The model under review builds one solid part; all positions refer to its coordinate system, in mm. A direction names the side the tool comes from. Round coordinates to 2 decimals unless told otherwise and drop trailing zeros. Write each loop counter-clockwise with the first axis right and the second up, starting at its lowest first coordinate (ties: lowest second). Pieces come first, ordered by that corner, then holes. Notation, with made-up numbers: (-35.5, 85.5) - (18.5, 85.5) arc R26 ccw to (18.5, 115.5) - close; hole circle Ø5 at (-9, -22). An arc over 180 degrees is marked (long way). Use one line per item in the form item = value.
Autodesk Inventor part; units mm, degrees
ref_plane "YZ Plane" through (0, 0, 0) normal (1, 0, 0) x (0, 1, 0)
ref_plane "XZ Plane" through (0, 0, 0) normal (0, 1, 0) x (-1, 0, 0)
ref_plane "XY Plane" through (0, 0, 0) normal (0, 0, 1) x (1, 0, 0)
sketch "Sketch2" plane through (0, 0, 0) normal (1, 0, 0) x (0, 1, 0)
  arc A0 (12.5, 50.9902) -> (-12.5, 50.9902) centre (0, 0) ccw
  arc A1 (-19.5, 39.443) -> (-17.7114, 42.7254) centre (-20.9403, 42.3564) ccw
  line L0 (-17.7114, 42.7254) -> (-17.7881, 43.3968)
  arc A2 (-12.5, 50.9902) -> (-17.7881, 43.3968) centre (-10.8333, 44.1915) ccw
  line L1 (0, 0) -> (0, 52.5) construction
  arc A3 (17.7114, 42.7254) -> (19.5, 39.443) centre (20.9403, 42.3564) ccw
  line L2 (17.7114, 42.7254) -> (17.7881, 43.3968)
  arc A4 (17.7881, 43.3968) -> (12.5, 50.9902) centre (10.8333, 44.1915) ccw
  arc A5 (-44.6318, 27.645) -> (-52.3573, 3.8686) centre (0, 0) ccw
  arc A6 (-43.5384, -6.357) -> (-46.1074, -3.6416) centre (-46.7543, -6.8266) ccw
  line L3 (-46.1074, -3.6416) -> (-46.7696, -3.5071)
  arc A7 (-52.3573, 3.8686) -> (-46.7696, -3.5071) centre (-45.3763, 3.3528) ccw
  line L4 (0, 0) -> (-49.9305, 16.2234) construction
  arc A8 (-35.776, 30.3278) -> (-44.6318, 27.645) centre (-38.6809, 23.959) ccw
  line L5 (-35.1611, 30.0474) -> (-35.776, 30.3278)
  arc A9 (-35.1611, 30.0474) -> (-31.4867, 30.7342) centre (-33.8124, 33.0043) ccw
  arc A10 (-40.084, -33.9046) -> (-19.8586, -48.5993) centre (0, 0) ccw
  arc A11 (-7.4082, -43.3719) -> (-10.7846, -44.976) centre (-7.9554, -46.5755) ccw
  line L6 (-10.7846, -44.976) -> (-11.1171, -45.5643)
  arc A12 (-19.8586, -48.5993) -> (-11.1171, -45.5643) centre (-17.2108, -42.1194) ccw
  line L7 (0, 0) -> (-30.8587, -42.4734) construction
  arc A13 (-39.8989, -24.6532) -> (-40.084, -33.9046) centre (-34.7395, -29.384) ccw
  line L8 (-39.4421, -24.1551) -> (-39.8989, -24.6532)
  arc A14 (-39.4421, -24.1551) -> (-38.9598, -20.4482) centre (-41.8376, -21.9586) ccw
  arc A15 (19.8586, -48.5993) -> (40.084, -33.9046) centre (0, 0) ccw
  arc A16 (38.9598, -20.4482) -> (39.4421, -24.1551) centre (41.8376, -21.9586) ccw
  line L9 (39.4421, -24.1551) -> (39.8989, -24.6532)
  arc A17 (40.084, -33.9046) -> (39.8989, -24.6532) centre (34.7395, -29.384) ccw
  line L10 (0, 0) -> (30.8587, -42.4734) construction
  arc A18 (11.1171, -45.5643) -> (19.8586, -48.5993) centre (17.2108, -42.1194) ccw
  line L11 (10.7846, -44.976) -> (11.1171, -45.5643)
  arc A19 (10.7846, -44.976) -> (7.4082, -43.3719) centre (7.9554, -46.5755) ccw
  arc A20 (52.3573, 3.8686) -> (44.6318, 27.645) centre (0, 0) ccw
  arc A21 (31.4867, 30.7342) -> (35.1611, 30.0474) centre (33.8124, 33.0043) ccw
  line L12 (35.1611, 30.0474) -> (35.776, 30.3278)
  arc A22 (44.6318, 27.645) -> (35.776, 30.3278) centre (38.6809, 23.959) ccw
  line L13 (0, 0) -> (49.9305, 16.2234) construction
  arc A23 (46.7696, -3.5071) -> (52.3573, 3.8686) centre (45.3763, 3.3528) ccw
  line L14 (46.1074, -3.6416) -> (46.7696, -3.5071)
  arc A24 (46.1074, -3.6416) -> (43.5384, -6.357) centre (46.7543, -6.8266) ccw
  arc A25 (38.9598, -20.4482) -> (43.5384, -6.357) centre (0, 0) ccw
  arc A26 (-7.4082, -43.3719) -> (7.4082, -43.3719) centre (0, 0) ccw
  arc A27 (-43.5384, -6.357) -> (-38.9598, -20.4482) centre (0, 0) ccw
  arc A28 (31.4867, 30.7342) -> (19.5, 39.443) centre (0, 0) ccw
  arc A29 (-19.5, 39.443) -> (-31.4867, 30.7342) centre (0, 0) ccw
  dimension "d75" = 52.5
  dimension "d76" = 7
  dimension "d77" = 3.25
  dimension "d80" = 360
  dimension "d83" = 44
  dimension "d84" = 12.5
  dimension "d85" = 19.5
extrude "Extrusion1" add sketch "Sketch2" along normal blind 5
sketch "Sketch3" plane through (0, 0, 0) normal (-1, 0, 0) x (0, 0, 1)
  circle A0 centre (0, 0) radius 11.5
  circle A1 centre (0, 0) radius 9
  point P0 (0, 0)
  dimension "d55" = 23
  dimension "d56" = 18
extrude "Extrusion2" add sketch "Sketch3" along normal blind 27.81
fillet "Fillet1" radius 14 1 edges at (0, 0, -11.5)
sketch "Sketch4" plane through (5, 0, 0) normal (1, 0, 0) x (0, 0, -1)
  circle A0 centre (0, 0) radius 32.5
  point P0 (0, 0)
  dimension "d60" = 65
extrude "Extrusion3" add sketch "Sketch4" along normal blind 5
sketch "Sketch5" plane through (10, 0, 0) normal (1, 0, 0) x (0, 0, -1)
  circle A0 centre (0, 0) radius 13
  point P0 (0, 0)
  dimension "d63" = 26
extrude "Extrusion4" add sketch "Sketch5" along normal blind 3.108
sketch "Sketch6" plane through (13.108, 0, 0) normal (1, 0, 0) x (0, 0, -1)
  circle A0 centre (0, 0) radius 9
  point P0 (0, 0)
extrude "Extrusion5" cut sketch "Sketch6" against normal through all
sketch "Sketch7" plane through (5, 0, 0) normal (1, 0, 0) x (0, 0, -1)
  circle A0 centre (-45, 0) radius 2.5
  point P0 (0, 0)
  dimension "d68" = 45
  dimension "d69" = 5
extrude "Extrusion6" cut sketch "Sketch7" against normal through all
pattern_circular "Circular Pattern1" count 5 over 360 about axis through (-10, 0, 0) along (1, 0, 0) of "Extrusion6"
properties part number "362-03"
(1) The part is to be moulded in two halves that separate along Y. For faces 4 (the cylindrical face through (11.532, 7.91, 10.316)), 5 (the cylindrical face through (2.465, -40.778, 30.637)), 6 (the cylindrical face through (2.46, -16.62, 48.13)), say which applies: +Y half, -Y half, draft (parallel to the pull), parting line (faces both ways), or undercut.
Geometry results:
face_4 = parting line
face_5 = undercut
face_6 = -Y half
(2) Add section A-A on y = -27. Write out the cut boundary in (x, z) (3 decimals), then the cut area to 3 significant figures.
Geometry results:
outline = (0, -45.025) - (5, -45.025) - (5, -38.845) - (0, -38.845) - close; (0, -33.967) - (5, -33.967) - (5, -18.09) - (10, -18.09) - (10, 18.09) - (5, 18.09) - (5, 34.742) - (0, 34.742) - close
area = 555 mm2
(3) Machinability: for faces 1 (the cylindrical face through (2.465, 41.879, -13.498)), 2 (the cylindrical face through (-20.8, -11.4, -1.5)), 3 (the flat face through (5, 23, 25)), which of the approach directions +Z, -Z, +X, -X, +Y, -Y give a long, thin tool a straight path to every point of the face, cutting with its end or side? Answer none if there is none.
Geometry results:
face_1 = +X, -X, +Y
face_2 = -X
face_3 = +X
(4) Add section B-B on z = 45. Write out the cut boundary in (x, y).
Geometry results:
outline = (0, -17.79) - (5, -17.79) - (5, -2.5) - (0, -2.5) - close; (0, 2.5) - (5, 2.5) - (5, 17.79) - (0, 17.79) - close
(5) To check wall thickness, follow L1, parallel to X at y = -20.5, z = -35.5; L2, parallel to Z at x = 4, y = -6; L3, parallel to Z at x = 6.5, y = 1. State the ranges of each line that lie inside material, in increasing order.
Geometry results:
L1 = 0 to 5
L2 = -43.59 to -6.71, 6.71 to 52.16
L3 = -32.48 to -8.94, 8.94 to 32.48
(6) Add section C-C on z = 0. Write out the cut boundary in (x, y), then the cut area to 3 significant figures.
Geometry results:
outline = (-27.81, -11.5) - (-14, -11.5) arc R14 cw to (0, -25.5) - (0, -51.52) - (5, -51.52) - (5, -32.5) - (10, -32.5) - (10, -13) - (13.11, -13) - (13.11, -9) - (-27.81, -9) - close; (-27.81, 9) - (13.11, 9) - (13.11, 13) - (10, 13) - (10, 32.5) - (5, 32.5) - (5, 51.52) - (0, 51.52) - (0, 25.5) arc R14 cw to (-14, 11.5) - (-27.81, 11.5) - close
area = 908 mm2
(7) Insertion check: P1, Ø6, axis at y = 26.45, z = -36.41, coming from the -X side; P2, Ø4.5, axis at y = 0, z = 45, coming from the +X side; P3, Ø8, axis at y = 42.8, z = 13.91, coming from the +X side; P4, Ø8, axis at x = -17.5, y = 11.5, coming from the -Z side. Each pin has a flat end and moves straight along its axis. Give the tip position at first contact, or say it passes through.
Geometry results:
P1 = 0
P2 = through
P3 = 5
P4 = -8.72
